```python
from build123d import *

# Parameters (mm, degrees)
SKETCH1_R           = 1.27
SKETCH1_W           = 30.48
SKETCH1_H           = 14.478
BOSS_EXTRUDE1_DEPTH = 4.4958


with BuildPart() as part:
    # Sketch1 → Boss-Extrude1 (new body)
    with BuildSketch(Plane(origin=(0, 0, 0), x_dir=(1, 0, 0), z_dir=(0, 1, 0))):
        with BuildLine():
            Line((-92.209627628, 24.227655619), (-15.255255255, 48.455311237))
            ThreePointArc((-15.255255255, 48.455311237), (0, 50.8), (15.255255255, 48.455311237))
            Line((15.255255255, 48.455311237), (92.209627628, 24.227655619))
            ThreePointArc((92.209627628, 24.227655619), (109.982, 0), (92.209627628, -24.227655619))
            Line((92.209627628, -24.227655619), (15.255255255, -48.455311237))
            ThreePointArc((15.255255255, -48.455311237), (0, -50.8), (-15.255255255, -48.455311237))
            Line((-15.255255255, -48.455311237), (-92.209627628, -24.227655619))
            ThreePointArc((-92.209627628, -24.227655619), (-109.982, 0), (-92.209627628, 24.227655619))
        make_face()
        with Locations(Location((-56.603365496, 28.780358137, 0), (0, 0, 270))):
            Circle(SKETCH1_R, mode=Mode.SUBTRACT)
        with Locations(Location((-56.603365496, -28.780358137, 0), (0, 0, 270))):
            Circle(SKETCH1_R, mode=Mode.SUBTRACT)
        with Locations(Location((56.603365496, -28.780358137, 0), (0, 0, 270))):
            Circle(SKETCH1_R, mode=Mode.SUBTRACT)
        with Locations(Location((56.603365496, 28.780358137, 0), (0, 0, 270))):
            Circle(SKETCH1_R, mode=Mode.SUBTRACT)
        with Locations(Location((-26.314105966, 38.316369233, 0), (0, 0, 270))):
            Circle(SKETCH1_R, mode=Mode.SUBTRACT)
        with Locations(Location((26.314105966, 38.316369233, 0), (0, 0, 270))):
            Circle(SKETCH1_R, mode=Mode.SUBTRACT)
        Rectangle(SKETCH1_W, SKETCH1_H, mode=Mode.SUBTRACT)
    extrude(amount=BOSS_EXTRUDE1_DEPTH)


solid = part.part
```
Input: part model. Units: mm. Frame: model coordinates. A direction names the side the tool comes from. Round coordinates to 2 decimals unless told otherwise and drop trailing zeros. Loops run counter-clockwise (first coordinate to the right, second up) from the corner with the lowest first, then second, coordinate; pieces in that order, holes last.
1) Pull-direction query (Z, two-part tool) for faces 3 (the flat face through (-53.194, 2.216, 36.511)), 4 (the flat face through (-15.24, 2, 0)), 5 (the flat face through (2, 0, 11)); classes: released by +Z, released by -Z, zero draft, split by the parting line, or undercut.
Ans:
face 3: released by +Z
face 4: undercut
face 5: zero draft
2) Section query B-B on y = 1.75. Return the cut outline in (x, z).
Ans:
outline: (-92.21, -24.23) - (-15.26, -48.46) arc R50.8 ccw to (15.26, -48.46) - (92.21, -24.23) arc R25.4 ccw to (92.21, 24.23) - (15.26, 48.46) arc R50.8 ccw to (-15.26, 48.46) - (-92.21, 24.23) arc R25.4 ccw to start; hole circle Ø2.54 at (-56.6, -28.78); hole circle Ø2.54 at (-56.6, 28.78); hole circle Ø2.54 at (-26.31, -38.32); hole (-15.24, -7.24) - (15.24, -7.24) - (15.24, 7.24) - (-15.24, 7.24) - close; hole circle Ø2.54 at (26.31, -38.32); hole circle Ø2.54 at (56.6, -28.78); hole circle Ø2.54 at (56.6, 28.78)
3) Set-up query: faces 1 (the flat face through (15.24, 2, 0)), 2 (the cylindrical face through (0.2, 2.2, 50.8)). Return all of +Z, -Z, +X, -X, +Y, -Y with unobstructed straight access to the full face (end or side cutting, diameter ignored); none if empty.
Ans:
face 1: +Y, -Y
face 2: +Z, +Y, -Y
4) Section query D-D on x = 66. Return the cut outline in (y, z).
Ans:
outline: (0, -32.48) - (4.5, -32.48) - (4.5, 32.48) - (0, 32.48) - close
5) Material intervals for line 1 (Z direction, x = 1.5, y = 2.5); line 2 (Z direction, x = 9, y = 1.25); line 3 (Z direction, x = 87, y = 1), sorted ascending.
Ans:
line 1: z = -50.78 to -7.24, 7.24 to 50.78
line 2: z = -50 to -7.24, 7.24 to 50
line 3: z = -25.87 to 25.87
6) Section query A-A on x = 9. Return the cut outline in (y, z), plus the area to 3 significant figures.
Ans:
outline: (0, -50) - (4.5, -50) - (4.5, -7.24) - (0, -7.24) - close; (0, 7.24) - (4.5, 7.24) - (4.5, 50) - (0, 50) - close
area: 384 mm2
7) Section query C-C on z = -20.5. Return the cut outline in (x, y).
Ans:
outline: (-99.58, 0) - (99.58, 0) - (99.58, 4.5) - (-99.58, 4.5) - close
8) Pin query (flat end, axial travel): pin 1 (2 mm diameter, centred on x = 3.5, y = 3, fed in from -Z); pin 2 (1.5 mm diameter, centred on x = -43, y = 2, fed in from +Z); pin 3 (1.5 mm diameter, centred on y = 3.5, z = 16, fed in from -X). Return the tip coordinate at first contact, or that it passes through.
Ans:
pin 1: stops at z = -50.74
pin 2: stops at z = 39.96
pin 3: stops at x = -104.89
